from build123d import *

# Parameters (mm, degrees)
BOSS_EXTRUDE1_DEPTH = 7
SKETCH4_R           = 2.75
CUT_EXTRUDE3_DEPTH  = 7
SKETCH6_R           = 2.5
CUT_EXTRUDE4_DEPTH  = 31
SKETCH7_R           = 4
CUT_EXTRUDE5_DEPTH  = 5
CHAMFER_1_SIZE      = 0.3
FILLET_1_R          = 0.2


with BuildPart() as part:
    # Sketch1 → Boss-Extrude1 (new body, symmetric)
    with BuildSketch(Plane(origin=(0, 0, 0), x_dir=(0, 0, -1), z_dir=(1, 0, 0))):
        with BuildLine():
            Line((-21, 0), (21, 0))
            Line((21, 0), (21, 6))
            Line((21, 6), (9, 6))
            Line((9, 6), (9, 32.8))
            Line((9, 32.8), (1, 32.8))
            Line((1, 32.8), (1, 23.872983346))
            ThreePointArc((1, 23.872983346), (0, 16), (-1, 23.872983346))
            Line((-1, 23.872983346), (-1, 32.8))
            Line((-1, 32.8), (-9, 32.8))
            Line((-9, 32.8), (-9, 6))
            Line((-9, 6), (-21, 6))
            Line((-21, 6), (-21, 0))
        make_face()
    extrude(amount=BOSS_EXTRUDE1_DEPTH, both=True)

    # Sketch4 → Cut-Extrude3 (cut, through all)
    with BuildSketch(Plane(origin=(0, 6, 0), x_dir=(1, 0, 0), z_dir=(0, 1, 0))):
        with Locations(Location((0, -16, 0), (0, 0, 270))):  # turned: the seam where the file's is
            Circle(SKETCH4_R)
        with Locations(Location((0, 16, 0), (0, 0, 270))):  # turned: the seam where the file's is
            Circle(SKETCH4_R)
    extrude(amount=-CUT_EXTRUDE3_DEPTH, mode=Mode.SUBTRACT)

    # Sketch6 → Cut-Extrude4 (cut, through all)
    with BuildSketch(Plane(origin=(0, 0, -9), x_dir=(-1, 0, 0), z_dir=(0, 0, -1))):
        with Locations(Location((0, 27.8, 0), (0, 0, 90))):  # turned: the seam where the file's is
            Circle(SKETCH6_R)
    extrude(amount=-CUT_EXTRUDE4_DEPTH, mode=Mode.SUBTRACT)

    # Sketch7 → Cut-Extrude5 (cut)
    with BuildSketch(Plane(origin=(0, 0, -9), x_dir=(-1, 0, 0), z_dir=(0, 0, -1))):
        with Locations(Location((0, 27.8, 0), (0, 0, 90))):  # turned: the seam where the file's is
            Circle(SKETCH7_R)
    extrude(amount=-CUT_EXTRUDE5_DEPTH, mode=Mode.SUBTRACT)

    # Фаска1
    chamfer_1_edges = [part.edges().sort_by_distance(p)[0] for p in [
        (-7, 16, 0),
        (7, 16, 0),
        (0, 0, 13.25),
        (0, 6, 13.25),
        (0, 0, -18.75),
        (0, 6, -18.75),
        (0, 25.3, 9),
        (0, 23.8, -9),
    ]]
    chamfer(chamfer_1_edges, length=CHAMFER_1_SIZE)

    # Скругление1
    fillet_1_edges = [part.edges().sort_by_distance(p)[0] for p in [
        (-7, 32.8, 5),
        (-7, 19.4, 9),
        (-7, 6, 15),
        (-7, 3, 21),
        (-7, 0, 0),
        (-7, 3, -21),
        (-7, 6, -15),
        (-7, 19.4, -9),
        (-7, 32.8, -5),
        (-7, 28.491052367, -1),
        (-7, 15.7, 0),
        (-7, 28.491052367, 1),
        (7, 32.8, -5),
        (7, 19.4, -9),
        (7, 6, -15),
        (7, 3, -21),
        (7, 0, 0),
        (7, 3, 21),
        (7, 6, 15),
        (7, 19.4, 9),
        (7, 32.8, 5),
        (7, 28.491052367, 1),
        (7, 15.7, 0),
        (7, 28.491052367, -1),
        (0, 0, 21),
        (0, 6, 9),
        (0, 6, 21),
        (0, 32.8, 9),
        (0, 0, -21),
        (0, 32.8, -9),
        (0, 6, -9),
        (0, 6, -21),
    ]]
    fillet(fillet_1_edges, radius=FILLET_1_R)


solid = part.part
Input: part model. Units: mm. Frame: model coordinates. A direction names the side the tool comes from. Coordinates: 2 decimals unless noted, no trailing zeros. Order: outer loops, then holes, each group sorted by start corner. A loop starts at its lowest first (then second) coordinate and runs counter-clockwise, first axis right, second up. Notation, with made-up numbers: M -3.75,-16 L 28.25,-16 A23 ccw 28.25,20 Z; hole C -36.75,-17 d3. An arc over 180 degrees is marked long. Answer in a Markdown table with one row per item.
(1) Draft query along X for faces 1 (the cylindrical face through (-1.532, 31.495, -6.383)), 2 (the flat face through (0, 32.8, -5)), 3 (the cylindrical face through (0.751, 30.185, -2.521)), 4 (the flat face through (-7, 13, -1)). Return one class per face: pulls with the +X half, pulls with the -X half, needs draft (parallel to the pull), parting line crosses it, or undercut.
Numbers:
| item | result |
|---|---|
| face 1 | undercut |
| face 2 | needs draft |
| face 3 | undercut |
| face 4 | pulls with the -X half |
(2) Contact query for flat-ended pins moving along their axis: pin 1 Ø3 at (x, y) = (0, 27.8) entering from +Z; pin 2 Ø5 at (x, z) = (2.5, 11) entering from +Y; pin 3 Ø4 at (x, y) = (2.5, 20) entering from +Z; pin 4 Ø5 at (x, y) = (3.5, 21) entering from -Z. Output: stop coordinate, or through.
Numbers:
| item | result |
|---|---|
| pin 1 | passes through |
| pin 2 | stops at y = 32.8 |
| pin 3 | stops at z = 9 |
| pin 4 | stops at z = -9 |
(3) Section query A-A, the plane z = 16. Output: boundary loops of the cut face in (x, y).
Numbers:
| item | result |
|---|---|
| outline | M -7,0.2 A0.2 ccw -6.8,0 L -3.05,0 L -2.75,0.3 L -2.75,5.7 L -3.05,6 L -6.8,6 A0.2 ccw -7,5.8 Z; M 2.75,0.3 L 3.05,0 L 6.8,0 A0.2 ccw 7,0.2 L 7,5.8 A0.2 ccw 6.8,6 L 3.05,6 L 2.75,5.7 Z |
(4) Section query C-C, the plane y = 27.8. Give the number of separate pieces and of enclosed holes in the cut face, plus the area to 3 significant figures.
Numbers:
| item | result |
|---|---|
| separate pieces | 4 |
| enclosed holes | 0 |
| area | 129 mm^2 |
(5) Material intervals for line 1 (X direction, y = 4.65, z = -16); line 2 (Z direction, x = -5.75, y = 29.5); line 3 (Z direction, x = -0.5, y = 20), sorted ascending. Write a range as [from, to].
Numbers:
| item | result |
|---|---|
| line 1 | x = [-7, -2.75], [2.75, 7] |
| line 2 | z = [-9, -1], [1, 9] |
| line 3 | z = [-9, -4], [4, 9] |
(6) Access query for faces 5 (the flat face through (0, 20, 9)), 6 (the flat face through (0, 16, -9)), 7 (the flat face through (2, 30, 1)), 8 (the cylindrical face through (0.121, 3.038, 13.253)). Directions: +Z, -Z, +X, -X, +Y, -Y. A direction counts if a zero-diameter tool reaches every point of the face in a straight line with its end or side. Return the directions, or none.
Numbers:
| item | result |
|---|---|
| face 5 | +Z, +X, -X, +Y |
| face 6 | -Z, +X, -X, +Y |
| face 7 | +X, -X, +Y |
| face 8 | +Y, -Y |
(7) Section query B-B, the plane y = 4.5. Output: boundary loops of the cut face in (x, z).
Numbers:
| item | result |
|---|---|
| outline | M -7,-20.8 A0.2 ccw -6.8,-21 L 6.8,-21 A0.2 ccw 7,-20.8 L 7,20.8 A0.2 ccw 6.8,21 L -6.8,21 A0.2 ccw -7,20.8 Z; hole C 0,-16 d5.5; hole C 0,16 d5.5 |
